from build123d import *

# Parameters (mm, degrees)
CROQUIS1_W              = 20
CROQUIS1_H              = 16
SALIENTE_EXTRUIR1_DEPTH = 2
SALIENTE_EXTRUIR2_DEPTH = 2
CROQUIS3_R              = 1
SALIENTE_EXTRUIR3_DEPTH = 3
SALIENTE_EXTRUIR4_DEPTH = 2


with BuildPart() as part:
    # Croquis1 → Saliente-Extruir1 (new body)
    with BuildSketch(Plane.XY):
        Rectangle(CROQUIS1_W, CROQUIS1_H)
    extrude(amount=SALIENTE_EXTRUIR1_DEPTH)

    # Croquis2 → Saliente-Extruir2 (add)
    with BuildSketch(Plane.XY.offset(2)):
        with BuildLine():
            Line((-1, -3.5), (-1, -8))
            Line((-1, -8), (1, -8))
            Line((1, -8), (1, -3.5))
            ThreePointArc((1, -3.5), (3.752648906, -1.325939397), (6.934939372, 0.149405611))
            ThreePointArc((6.934939372, 0.149405611), (8.874367576, 3.859075687), (5.217391304, 5.896122171))
            ThreePointArc((5.217391304, 5.896122171), (0, 5.203603311), (-5.217391304, 5.896122171))
            ThreePointArc((-5.217391304, 5.896122171), (-8.874367576, 3.859075687), (-6.934939372, 0.149405611))
            ThreePointArc((-6.934939372, 0.149405611), (-3.752648906, -1.325939397), (-1, -3.5))
        make_face()
    extrude(amount=SALIENTE_EXTRUIR2_DEPTH)

    # Croquis3 → Saliente-Extruir3 (add)
    with BuildSketch(Plane.XY.offset(4)):
        with Locations((-6, 3)):
            Circle(CROQUIS3_R)
        with Locations((6, 3)):
            Circle(CROQUIS3_R)
    extrude(amount=SALIENTE_EXTRUIR3_DEPTH)

    # Croquis5 → Saliente-Extruir4 (add)
    with BuildSketch(Plane.ZY.offset(1)):
        with BuildLine():
            Line((4, -8), (2, -8))
            ThreePointArc((2, -8), (11, -17), (20, -8))
            ThreePointArc((20, -8), (19, -7), (18, -8))
            ThreePointArc((18, -8), (11, -15), (4, -8))
        make_face()
    extrude(amount=-SALIENTE_EXTRUIR4_DEPTH)


solid = part.part
Here's how the part is built. I have some questions about the finished solid (model axes, mm). A direction names the side the tool comes from. Give positions to 0.01 mm unless a question says otherwise; leave off trailing zeros. Write each loop counter-clockwise with the first axis right and the second up, starting at its lowest first coordinate (ties: lowest second). Pieces come first, ordered by that corner, then holes. Notation, with made-up numbers: (-28, 81.25) -> (-11, 81.25) arc R17 cw to (-11, 103.25) -> close; hole circle Ø10 at (5.5, -3.5). An arc over 180 degrees is marked (long way). Use one line per item in the form item = value. Start each with the question number.
1. Imagine slicing it at D-D on x = -6. List the corners of the cut face in (y, z) for me.
2. Imagine slicing it at B-B on z = 4.75. List the corners of the cut face in (x, y) for me.
3. Imagine slicing it at C-C on y = -14. List the corners of the cut face in (x, z) for me.
4. On a 3-axis mill with a long thin cutter (end or side, diameter ignored), from which of +Z, -Z, +X, -X, +Y, -Y can I reach the whole of each face in a straight line? I mean faces 1 (the face through (5, 3, 5)), 2 (the face through (-3.795, -1.3, 2.986)), 3 (the face through (-6, 3, 7)), 4 (the face through (1, -15, 9)), 5 (the face through (0.074, 5.204, 2.986)). Say none if no direction works.
5. Imagine slicing it at A-A on y = -6. List the corners of the cut face in (x, z) for me.
6. Thinking about a two-plate mould opening in Z: for faces 6 (the face through (-2, -3, 2)), 7 (the face through (0, 8, 1)), 8 (the face through (0, -7, 19)), which applies, +Z half, -Z half, draft (parallel to the pull), parting line (faces both ways), or undercut?
7. If I drill on L1, parallel to Z at x = 5.75, y = 4.75; L2, parallel to X at y = -6.25, z = 3; L3, parallel to Z at x = 5.25, y = -5, over which ranges is the centre line in solid material (lowest first)?
8. Will these pins go through, and if not, where does the flat tip stop? pin 1 Ø2 at (x, z) = (0.5, 2.5) entering from -Y; pin 2 Ø1.6 at (x, y) = (5.5, 3) entering from +Z; pin 3 Ø0.6 at (x, z) = (-1, 1) entering from -Y.
Entries:
q1.outline = (-8, 0) -> (8, 0) -> (8, 2) -> (6, 2) -> (6, 4) -> (4, 4) -> (4, 7) -> (2, 7) -> (2, 4) -> (-0.19, 4) -> (-0.19, 2) -> (-8, 2) -> close
q2.outline = circle Ø2 at (-6, 3); (-1, -14.48) -> (1, -14.48) -> (1, -11.15) -> (-1, -11.15) -> close; circle Ø2 at (6, 3)
q3.outline = (-1, 4.29) -> (1, 4.29) -> (1, 7.39) -> (-1, 7.39) -> close; (-1, 14.61) -> (1, 14.61) -> (1, 17.71) -> (-1, 17.71) -> close
q4.face_1 = +Z
q4.face_2 = +Z, -X, -Y
q4.face_3 = +Z, +X, -X, +Y, -Y
q4.face_4 = +Z, +X, -Y
q4.face_5 = +Z, +Y
q5.outline = (-10, 0) -> (10, 0) -> (10, 2) -> (1, 2) -> (1, 4) -> (-1, 4) -> (-1, 2) -> (-10, 2) -> close
q6.face_6 = +Z half
q6.face_7 = draft
q6.face_8 = undercut
q7.L1 = 0 to 4
q7.L2 = -1 to 1
q7.L3 = 0 to 2
q8.pin_1 = -12.97
q8.pin_2 = 7
q8.pin_3 = -8
